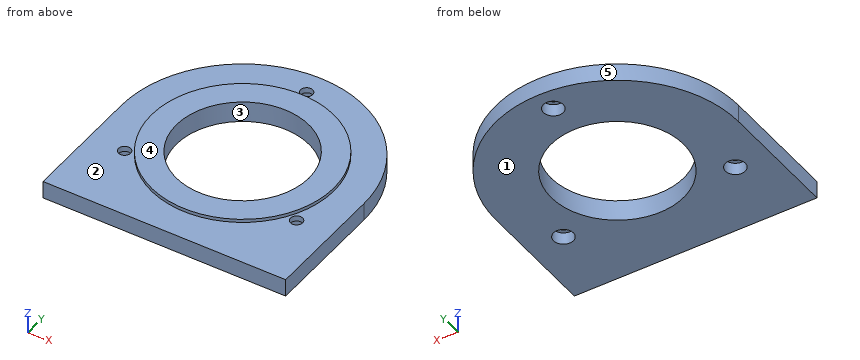
```python
from build123d import *

# Parameters (mm, degrees)
SKETCH_1_R                = 110
EXTRUDE_1_DEPTH           = 16
SKETCH_2_W                = 220
SKETCH_2_H                = 110
EXTRUDE_2_DEPTH           = 16
SKETCH_3_R                = 82.5
EXTRUDE_3_DEPTH           = 3
HOLE_WIZARD_1_D           = 11
HOLE_WIZARD_1_CBORE_D     = 18
HOLE_WIZARD_1_CBORE_DEPTH = 11
PATTERN_CIRCULAR_1_COUNT  = 3
SKETCH_6_R                = 60
CUT_EXTRUDE_1_DEPTH       = 157.719494639


with BuildPart() as part:
    # 草图1 → 凸台-拉伸1 (new body)
    with BuildSketch(Plane.XY):
        Circle(SKETCH_1_R)
    extrude(amount=EXTRUDE_1_DEPTH)

    # 草图2 → 凸台-拉伸2 (add)
    with BuildSketch(Plane.XY.offset(16)):
        with Locations((0, -55)):
            Rectangle(SKETCH_2_W, SKETCH_2_H)
    extrude(amount=-EXTRUDE_2_DEPTH)

    # 草图3 → 凸台-拉伸3 (add)
    with BuildSketch(Plane.XY.offset(16)):
        Circle(SKETCH_3_R)
    extrude(amount=EXTRUDE_3_DEPTH)

    # 打孔尺寸(%根据)内六角圆柱头螺钉的类型1 (through all)
    with Locations(Plane(origin=(0, 0, 0), x_dir=(-1, 0, 0), z_dir=(0, 0, -1))):
        with Locations((0, 90)):
            hole_wizard_1 = CounterBoreHole(HOLE_WIZARD_1_D / 2, HOLE_WIZARD_1_CBORE_D / 2, HOLE_WIZARD_1_CBORE_DEPTH)

    # 阵列(圆周)1: 打孔尺寸(%根据)内六角圆柱头螺钉的类型1 ×3 about axis
    pattern_circular_1_axis = Axis((0, 0, 0), (0, 0, 1))
    for i in range(1, PATTERN_CIRCULAR_1_COUNT):
        add(hole_wizard_1.rotate(pattern_circular_1_axis, i * 360 / PATTERN_CIRCULAR_1_COUNT), mode=Mode.SUBTRACT)

    # 草图6 → 切除-拉伸1 (cut, through all)
    with BuildSketch(Plane(origin=(0, 0, 0), x_dir=(-1, 0, 0), z_dir=(0, 0, -1))):
        Circle(SKETCH_6_R)
    extrude(amount=-CUT_EXTRUDE_1_DEPTH, mode=Mode.SUBTRACT)


solid = part.part
```
Could you check a few things on this model? Use its own coordinates, in mm. Face numbers are marked on the shaded views. A direction names the side the tool comes from. Round coordinates to 2 decimals unless told otherwise and drop trailing zeros. Loops run counter-clockwise (first coordinate to the right, second up) from the corner with the lowest first, then second, coordinate; pieces in that order, holes last. Notation, with made-up numbers: (53, 51.5) - (102, 51.5) arc R16 ccw to (102, 67.5) - close; hole circle Ø6 at (29, 75.25). An arc over 180 degrees is marked (long way). Answer in a Markdown table with one row per item. Add a question column.
(1) If we section it at A-A (x = 0): Please give me the cut outline in (y, z), plus the area to 3 significant figures.
(2) If we section it at B-B (y = 45.5): Please give me the cut outline in (x, z).
(3) For the marked faces 1 and 2, which set-ups out of +Z, -Z, +X, -X, +Y, -Y let a thin tool reach every point of the face, with its end or its side?
(4) If we section it at D-D (y = -45): Please give me the cut outline in (x, z).
(5) If we mould it in two halves opening along Y, with no side actions, what happens to the marked faces 3, 4 and 5? For each: pulls with the +Y half, pulls with the -Y half, needs draft (parallel to the pull), parting line crosses it, or undercut.
(6) I'm going to push flat-ended pins straight in: pin 1 (1.5 mm diameter, centred on x = -42, z = 6, fed in from +Y); pin 2 (2 mm diameter, centred on y = 43, z = 6, fed in from -X); pin 3 (14.5 mm diameter, centred on x = 77.94, y = -45, fed in from +Z); pin 4 (20 mm diameter, centred on x = -78.5, y = -42, fed in from -Z). Where does each tip first touch, or does it pass through?
(7) I need wall thicknesses on line 1 along Y through (x, z) = (0, 14.1); line 2 along Y through (x, z) = (0, 4.75); line 3 along X through (y, z) = (-49.5, 15.75). Which ranges of each line are inside material? Lowest first, please.
(8) If we section it at C-C (x = -27.5): Please give me the cut outline in (y, z), plus the area to 3 significant figures.
Model answer:
| question | item | result |
|---|---|---|
| 1 | outline | (-110, 0) - (-60, 0) - (-60, 19) - (-82.5, 19) - (-82.5, 16) - (-110, 16) - close; (60, 0) - (81, 0) - (81, 11) - (84.5, 11) - (84.5, 16) - (82.5, 16) - (82.5, 19) - (60, 19) - close; (95.5, 11) - (99, 11) - (99, 0) - (110, 0) - (110, 16) - (95.5, 16) - close |
| 1 | area | 1,480 mm² |
| 2 | outline | (-100.15, 0) - (-39.11, 0) - (-39.11, 19) - (-68.82, 19) - (-68.82, 16) - (-100.15, 16) - close; (39.11, 0) - (100.15, 0) - (100.15, 16) - (68.82, 16) - (68.82, 19) - (39.11, 19) - close |
| 3 | face 1 | -Z, +X, -X, +Y, -Y |
| 3 | face 2 | +Z |
| 4 | outline | (-110, 0) - (-86.94, 0) - (-86.94, 11) - (-83.44, 11) - (-83.44, 16) - (-110, 16) - close; (-72.44, 11) - (-68.94, 11) - (-68.94, 0) - (-39.69, 0) - (-39.69, 19) - (-69.15, 19) - (-69.15, 16) - (-72.44, 16) - close; (39.69, 0) - (68.94, 0) - (68.94, 11) - (72.44, 11) - (72.44, 16) - (69.15, 16) - (69.15, 19) - (39.69, 19) - close; (83.44, 11) - (86.94, 11) - (86.94, 0) - (110, 0) - (110, 16) - (83.44, 16) - close |
| 5 | face 3 | undercut |
| 5 | face 4 | needs draft |
| 5 | face 5 | pulls with the +Y half |
| 6 | pin 1 | stops at y = 101.97 |
| 6 | pin 2 | stops at x = -101.67 |
| 6 | pin 3 | stops at z = 16 |
| 6 | pin 4 | stops at z = 0 |
| 7 | line 1 | y = -110 to -60, 60 to 84.5, 95.5 to 110 |
| 7 | line 2 | y = -110 to -60, 60 to 81, 99 to 110 |
| 7 | line 3 | x = -110 to -81.1, -74.78 to -33.91, 33.91 to 74.78, 81.1 to 110 |
| 8 | outline | (-110, 0) - (-53.33, 0) - (-53.33, 19) - (-77.78, 19) - (-77.78, 16) - (-110, 16) - close; (53.33, 0) - (106.51, 0) - (106.51, 16) - (77.78, 16) - (77.78, 19) - (53.33, 19) - close |
| 8 | area | 1,900 mm² |
